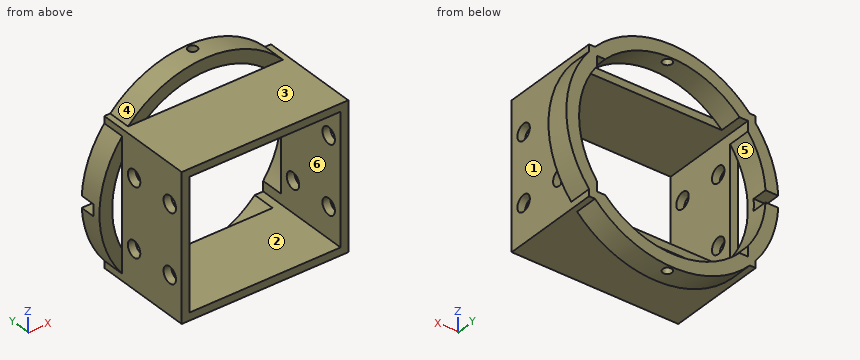
from build123d import *

# Parameters (mm, degrees)
F0_W      = 54.864
F0_H      = 47.752
F1_DEPTH  = 33.02
F2_W      = 24.892
F2_H      = 21.336
F3_DEPTH  = 33.02
F4_R      = 34.925
F4_R_2    = 30.734
F5_DEPTH  = 7.62
F6_R      = 2.6543
F7_DEPTH  = 76.2
F9_DEPTH  = 7.62
F11_DEPTH = 25.4
F12_R     = 30.734
F13_DEPTH = 7.62
F15_DEPTH = 5.08
F17_R     = 1.5113
F18_DEPTH = 127


with BuildPart() as f1:
    # F0 (on Front) → F1 (new body)
    with BuildSketch(Plane.XZ):
        Rectangle(F0_W, F0_H)
    extrude(amount=F1_DEPTH)

    # F2 (on face) → F3 (cut)
    with BuildSketch(Plane.XZ.offset(33.02)):
        with Locations((-12.446, 10.668)):
            Rectangle(F2_W, F2_H)
        with Locations((12.446, -10.668)):
            Rectangle(F2_W, F2_H)
        with Locations((-12.446, -10.668)):
            Rectangle(F2_W, F2_H)
        with Locations((12.446, 10.668)):
            Rectangle(F2_W, F2_H)
    extrude(amount=-F3_DEPTH, mode=Mode.SUBTRACT)

    # F4 (on face) → F5 (join)
    with BuildSketch(Plane(origin=(0, 0, 0), x_dir=(-1, 0, 0), z_dir=(0, 1, 0))):
        Circle(F4_R)
        Circle(F4_R_2, mode=Mode.SUBTRACT)
    extrude(amount=-F5_DEPTH)

    # F6 (on face) → F7 (cut)
    with BuildSketch(Plane.YZ.offset(27.432)):
        with Locations((-27.94, 11.176)):
            Circle(F6_R)
        with Locations((-27.94, -11.176)):
            Circle(F6_R)
        with Locations((-12.7, 11.176)):
            Circle(F6_R)
        with Locations((-12.7, -11.176)):
            Circle(F6_R)
    extrude(amount=-F7_DEPTH, mode=Mode.SUBTRACT)

    # F8 (on face) → F9 (join)
    with BuildSketch(Plane(origin=(0, 0, 0), x_dir=(-1, 0, 0), z_dir=(0, 1, 0))):
        Polygon((-15.239977, 28.93018), (-21.844286, 22.671998), (22.174528, 22.671998), (17.10213, 27.676882), (0, 33.06745), align=None)
        Polygon((-26.720829, -17.021414), (-26.720829, 16.84154), (-31.688731, 8.959086), (-33.177566, -3.639529), align=None)
        Polygon((-18.059891, -29.893076), (0, -33.054188), (13.156982, -30.942233), (22.121344, -22.471936), (-24.892, -22.471936), align=None)
        Polygon((26.667995, 16.763607), (26.667995, -17.988142), (32.70267, -7.179345), (32.70267, 5.721464), align=None)
    extrude(amount=-F9_DEPTH)

    # F10 (on face) → F11 (cut)
    with BuildSketch(Plane(origin=(0, 0, 0), x_dir=(-1, 0, 0), z_dir=(0, 1, 0))):
        Polygon((24.892, 21.336), (-22.121344, 21.336), (-24.892, 21.336), (-24.892, -18.026844), (-24.892, -21.336), (24.892, -21.336), align=None)
    extrude(amount=-F11_DEPTH, mode=Mode.SUBTRACT)

    # F12 (on face) → F13 (cut)
    with BuildSketch(Plane(origin=(0, 0, 0), x_dir=(-1, 0, 0), z_dir=(0, 1, 0))):
        Circle(F12_R)
    extrude(amount=-F13_DEPTH, mode=Mode.SUBTRACT)

    # F14 (on face) → F15 (cut)
    with BuildSketch(Plane(origin=(0, 0, 0), x_dir=(-1, 0, 0), z_dir=(0, 1, 0))):
        Polygon((34.873007, 1.905), (30.674904, 1.905), (30.031135, 1.905), (29.740494, -1.788886), (30.5029, -1.905), (30.674904, -1.905), (34.873007, -1.905), (38.508706, 0.957784), align=None)
    extrude(amount=-F15_DEPTH, mode=Mode.SUBTRACT)

    # F17 (on offset) → F18 (cut)
    with BuildSketch(Plane.XY.offset(76.2)):
        with Locations((0, -2.1463)):
            Circle(F17_R)
    extrude(amount=-F18_DEPTH, mode=Mode.SUBTRACT)


solid = f1.part
Verification items for the finished model (mm, model axes). Face numbers are marked on the shaded views. A direction names the side the tool comes from. Give positions to 0.01 mm unless a question says otherwise; leave off trailing zeros. Loops run counter-clockwise (first coordinate to the right, second up) from the corner with the lowest first, then second, coordinate; pieces in that order, holes last.
1) Set-up check for the marked faces 4, 5 and 6: record each of +Z, -Z, +X, -X, +Y, -Y from which the full face is reachable in a straight line by a thin tool's end or side.
2) Sectioned sample at A-A, the plane y = -12.7. Enter the section's corners in (x, z).
3) Sectioned sample at B-B, the plane x = 0. Enter the section's corners in (y, z) (3 decimals).
4) Sectioned sample at D-D, the plane z = 4. Enter the section's corners in (x, y).
5) Sectioned sample at C-C, the plane z = -28.5. Enter the section's corners in (x, y).
6) Depth check by flat-ended pin: pin 1 Ø8 at (x, z) = (5, -20.5) entering from +Y; pin 2 Ø1.1 at (x, z) = (-33, -0.5) entering from +Y; pin 3 Ø8.5 at (y, z) = (-27.94, 11.176) entering from -X; pin 4 Ø5 at (x, y) = (0, -2.15) entering from +Z (3 decimals). Enter the tip coordinate at first touch or a pass-through.
7) Thickness scan on line 1 along Z through (x, y) = (11, -27.5); line 2 along Z through (x, y) = (26.3, -27.94); line 3 along X through (y, z) = (-24, 12). Record the ranges inside material, lowest first.
8) Draft check along X on the marked faces 1, 2 and 3. Enter one of: pulls with the +X half, pulls with the -X half, needs draft (parallel to the pull), parting line crosses it, or undercut.
Answers:
1. face 4: +Z, +Y, -Y
1. face 5: +Y
1. face 6: +Y, -Y
2. outline: (-27.43, -23.88) - (27.43, -23.88) - (27.43, -13.83) - (24.89, -13.83) - (24.89, -21.34) - (-24.89, -21.34) - (-24.89, -13.83) - (-27.43, -13.83) - close; (-27.43, -8.52) - (-24.89, -8.52) - (-24.89, 8.52) - (-27.43, 8.52) - close; (-27.43, 13.83) - (-24.89, 13.83) - (-24.89, 21.34) - (24.89, 21.34) - (24.89, 13.83) - (27.43, 13.83) - (27.43, 23.88) - (-27.43, 23.88) - close; (24.89, -8.52) - (27.43, -8.52) - (27.43, 8.52) - (24.89, 8.52) - close
3. outline: (-33.02, -23.876) - (-7.62, -23.876) - (-7.62, -21.336) - (-33.02, -21.336) - close; (-33.02, 21.336) - (-7.62, 21.336) - (-7.62, 23.876) - (-33.02, 23.876) - close; (-7.62, -34.925) - (-3.658, -34.925) - (-3.658, -30.734) - (-7.62, -30.734) - close; (-7.62, 30.734) - (-3.658, 30.734) - (-3.658, 34.925) - (-7.62, 34.925) - close; (-0.635, -34.925) - (0, -34.925) - (0, -30.734) - (-0.635, -30.734) - close; (-0.635, 30.734) - (0, 30.734) - (0, 34.925) - (-0.635, 34.925) - close
4. outline: (-34.7, -7.62) - (-30.47, -7.62) - (-30.47, 0) - (-34.7, 0) - close; (-27.43, -33.02) - (-24.89, -33.02) - (-24.89, -7.62) - (-27.43, -7.62) - close; (24.89, -33.02) - (27.43, -33.02) - (27.43, -7.62) - (24.89, -7.62) - close; (30.47, -7.62) - (34.7, -7.62) - (34.7, 0) - (30.47, 0) - close
5. outline: (-20.19, -7.62) - (-11.5, -7.62) - (-11.5, 0) - (-20.19, 0) - close; (11.5, -7.62) - (20.19, -7.62) - (20.19, 0) - (11.5, 0) - close
6. pin 1: stops at y = -7.62
6. pin 2: stops at y = -5.08
6. pin 3: stops at x = -27.43
6. pin 4: stops at z = 34.925
7. line 1: z = -23.88 to -21.34, 21.34 to 23.88
7. line 2: z = -23.88 to -13.83, -8.52 to 8.52, 13.83 to 23.88
7. line 3: x = -27.43 to -24.89, 24.89 to 27.43
8. face 1: pulls with the +X half
8. face 2: undercut
8. face 3: needs draft
